Geometry check sheet. Reference: the model listing, model coordinates, mm. Face numbers are marked on the shaded views. A direction names the side the tool comes from. Coordinates: 2 decimals unless noted, no trailing zeros. Write each loop counter-clockwise with the first axis right and the second up, starting at its lowest first coordinate (ties: lowest second). Pieces come first, ordered by that corner, then holes.
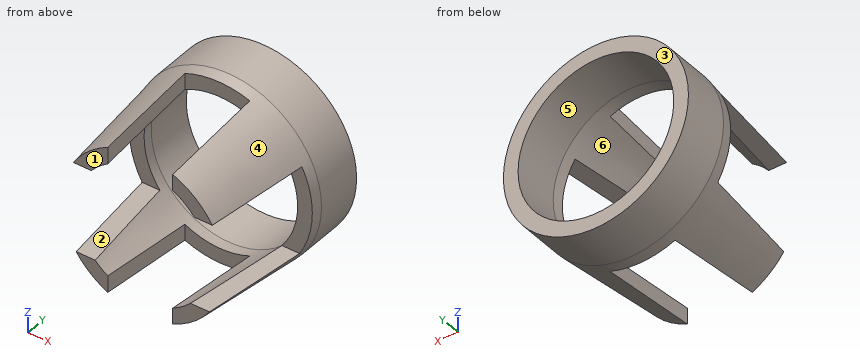
from build123d import *

# Parameters (mm, degrees)
F0_R           = 26.44775
F1_DEPTH       = 55.4101
F2_SIZE2       = 39.37
F2_SIZE        = 3.81
F3_R           = 31.4325
F4_DEPTH       = 55.4101
F5_SIZE2       = 39.37
F5_SIZE        = 3.81
F7_W           = 10.4550290853
F7_H           = 15.8277489245
F7_H_2         = 14.3756624311
F8_DEPTH       = 43.9235
F8_DEPTH_BACK  = 42.42753
F9_W           = 22.0717256889
F9_H           = 9.8741929978
F9_H_2         = 31.5537750721
F10_DEPTH      = 52.69923
F10_DEPTH_BACK = 50.37589


with BuildPart() as f1:
    # F0 (on Front) → F1 (new body)
    with BuildSketch(Plane.XZ):
        Circle(F0_R)
    extrude(amount=F1_DEPTH)

    # F2
    f2_edges = [f1.edges().sort_by_distance(p)[0] for p in [
        (-26.44775, -55.4101, 0),
    ]]
    f2_side = f1.faces().sort_by_distance((0, -55.4101, 0))[0]
    chamfer(f2_edges, length=F2_SIZE, length2=F2_SIZE2, reference=f2_side)


with BuildPart() as f4:
    # F3 (on Front) → F4 (new body)
    with BuildSketch(Plane.XZ):
        Circle(F3_R)
    extrude(amount=F4_DEPTH)

    # F5
    f5_edges = [f4.edges().sort_by_distance(p)[0] for p in [
        (-31.4325, -55.4101, 0),
    ]]
    f5_side = f4.faces().sort_by_distance((0, -55.4101, 0))[0]
    chamfer(f5_edges, length=F5_SIZE, length2=F5_SIZE2, reference=f5_side)

    # F6: cut F1
    add(f1.part, mode=Mode.SUBTRACT)

    # F7 (on Right) → F8 (cut, two sides)
    with BuildSketch(Plane.YZ) as f8_sk:
        with Locations((-24.9758986756, -7.9138744622)):
            Rectangle(F7_W, F7_H)
        with Locations((-24.9758986756, 7.1878312156)):
            Rectangle(F7_W, F7_H_2)
        Polygon((-30.2034132183, -15.8277489245), (-30.2034132183, 0), (-30.2034132183, 14.3756624311), (-65.0081411004, 14.3756624311), (-65.0081411004, -15.8277489245), align=None)
    extrude(amount=F8_DEPTH, mode=Mode.SUBTRACT)
    extrude(f8_sk.sketch, amount=-F8_DEPTH_BACK, mode=Mode.SUBTRACT)

    # F9 (on Top) → F10 (cut, two sides)
    with BuildSketch(Plane.XY) as f10_sk:
        with Locations((-0.8712508716, -25.1211086288)):
            Rectangle(F9_W, F9_H)
        with Locations((-0.8712508716, -45.8350926638)):
            Rectangle(F9_W, F9_H_2)
    extrude(amount=F10_DEPTH, mode=Mode.SUBTRACT)
    extrude(f10_sk.sketch, amount=-F10_DEPTH_BACK, mode=Mode.SUBTRACT)


solid = f4.part
1. Sectioned sample at D-D, the plane y = -7. Record the boundary of the cut face in (x, z) (1 decimal), and give its area (3 significant figures).
Computed values:
outline: circle Ø62.9 at (0, 0); hole circle Ø52.9 at (0, 0)
area: 906 mm2
2. Thickness scan on line 1 along X through (y, z) = (-5, 0.5); line 2 along Z through (x, y) = (0, -4); line 3 along Z through (x, y) = (-9, -3). Record the ranges inside material, lowest first.
Computed values:
line 1: x = -31.43 to -26.44, 26.44 to 31.43
line 2: z = -31.43 to -26.45, 26.45 to 31.43
line 3: z = -30.12 to -24.87, 24.87 to 30.12
3. Draft check along X on the marked faces 3, 4, 5 and 6. Enter one of: released by +X, released by -X, zero draft, split by the parting line, or undercut.
Computed values:
face 3: zero draft
face 4: split by the parting line
face 5: undercut
face 6: undercut
4. Gauge pin test, flat ends, axial feed: pin 1 Ø3 at (y, z) = (-29.5, -23) entering from +X; pin 2 Ø11.5 at (x, z) = (24, 1) entering from -Y; pin 3 Ø11 at (x, y) = (-22, -45.5) entering from -Z. Record the tip position at first contact, or that the pin passes through.
Computed values:
pin 1: stops at x = 21.12
pin 2: stops at y = -19.75
pin 3: stops at z = -23.39
5. Sectioned sample at B-B, the plane y = -46. Record the boundary of the cut face in (x, z), and give its area (3 significant figures).
Computed values:
outline: (-24.65, 14.38) - (-18.65, 14.38) arc R23.55 cw to (-11.91, 20.32) - (-11.91, 25.93) arc R28.53 ccw to start; (-23.74, -15.83) arc R28.53 ccw to (-11.91, -25.93) - (-11.91, -20.32) arc R23.55 cw to (-17.44, -15.83) - close; (10.16, -26.66) arc R28.53 ccw to (23.74, -15.83) - (17.44, -15.83) arc R23.55 cw to (10.16, -21.24) - close; (10.16, 21.24) arc R23.55 cw to (18.65, 14.38) - (24.65, 14.38) arc R28.53 ccw to (10.16, 26.66) - close
area: 266 mm2
6. Sectioned sample at A-A, the plane z = 0. Record the boundary of the cut face in (x, y), and give its area (3 significant figures).
Computed values:
outline: (-31.43, -16.04) - (-31.07, -19.75) - (-26.09, -19.75) - (-26.45, -16.04) - (-26.45, 0) - (-31.43, 0) - close; (26.09, -19.75) - (31.07, -19.75) - (31.43, -16.04) - (31.43, 0) - (26.45, 0) - (26.45, -16.04) - close
area: 197 mm2
7. Access from +Z, -Z, +X, -X, +Y, -Y to the whole of each face (thin tool, end or side, straight path). Record for the marked faces 1 and 2.
Computed values:
face 1: +Z, -Z, +X, -X, -Y
face 2: +X, -X, -Y
8. Sectioned sample at C-C, the plane x = 0. Record the boundary of the cut face in (y, z).
Computed values:
outline: (-20.18, -31.03) - (-16.04, -31.43) - (0, -31.43) - (0, -26.45) - (-16.04, -26.45) - (-20.18, -26.05) - close; (-20.18, 26.05) - (-16.04, 26.45) - (0, 26.45) - (0, 31.43) - (-16.04, 31.43) - (-20.18, 31.03) - close
